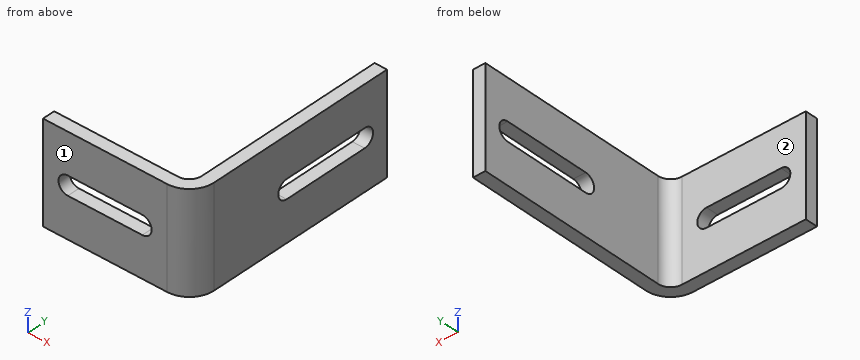
Autodesk Inventor part; units mm, degrees
ref_plane "YZ Plane" through (0, 0, 0) normal (1, 0, 0) x (0, 1, 0)
ref_plane "XZ Plane" through (0, 0, 0) normal (0, 1, 0) x (-1, 0, 0)
ref_plane "XY Plane" through (0, 0, 0) normal (0, 0, 1) x (1, 0, 0)
sketch "スケッチ1" plane through (0, 0, 0) normal (0, 1, 0) x (-1, 0, 0)
  line L0 (-10, 8) -> (10, 8)
  line L1 (10, 8) -> (10, -8)
  line L2 (10, -8) -> (-10, -8)
  line L3 (-10, -8) -> (-10, 8)
  line L4 (-10, 8) -> (10, -8) construction
  line L5 (10, 8) -> (-10, -8) construction
  point P0 (0, 0)
  dimension "d0" = 20
  dimension "d1" = 16
extrude "プレート1" add sketch "スケッチ1" along normal blind 2
sketch "スケッチ2" plane through (12, 4, -8) normal (1, 0, 0) x (0, 1, 0)
  line L0 (0, 16) -> (0, 0)
  line L1 (0, 0) -> (31, 0)
  line L2 (31, 0) -> (31, 16)
  line L3 (31, 16) -> (0, 16)
edge flange "フランジ1" height 35 angle 90 thickness 2 bend radius 2 thickness toward (1, 0, 0) relief tear relief width 2 relief depth 1 edges at (10, 2, 0) wall of the first edge with corners at (12, 4, 8) (12, 4, -8) (12, 35, -8) (12, 35, 8)
bend "曲げ1"
corner "コーナー1"
sketch "スケッチ3" plane through (14, 35, 8) normal (1, 0, 0) x (0, 0, -1)
  line L0 (6.5, -4) -> (6.5, -18)
  arc A0 (6.5, -18) -> (9.5, -18) centre (8, -18) ccw
  line L1 (9.5, -18) -> (9.5, -4)
  arc A1 (9.5, -4) -> (6.5, -4) centre (8, -4) ccw
  line L2 (16, 0) -> (16, -31)
  line L3 (0, 0) -> (16, 0)
  point P0 (8, -35)
  point P1 (8, 0)
  dimension "d19" = 1.5
extrude "押し出し1" cut sketch "スケッチ3" against normal blind 10
sketch "スケッチ4" plane through (0, 2, 0) normal (0, 1, 0) x (1, 0, 0)
  line L0 (-6, -1.5) -> (6, -1.5)
  arc A0 (6, -1.5) -> (6, 1.5) centre (6, 0) ccw
  line L1 (6, 1.5) -> (-6, 1.5)
  arc A1 (-6, 1.5) -> (-6, -1.5) centre (-6, 0) ccw
  line L2 (-10, -8) -> (-10, 8)
  line L3 (10, 8) -> (10, -8)
  point P0 (0, 0)
  dimension "d23" = 4
  dimension "d24" = 4
  dimension "d25" = 1.5
extrude "押し出し2" cut sketch "スケッチ4" against normal blind 10
equation "\"d2\" = Thickness"
equation "\"d3\" = BendReliefWidth"
equation "\"d4\" = BendReliefDepth"
equation "\"d5\" = MinimumRemnant"
equation "\"d6\" = TransitionRadius"
equation "\"d9\" = BendRadius"
equation "\"d10\" = CornerReliefSize"
equation "\"d11\" = GapSize"
equation "\"d12\" = JacobiRadiusSize"
equation "\"BendRadius\" = Thickness"
equation "\"BendReliefWidth\" = Thickness"
equation "\"BendReliefDepth\" = 0.5 * Thickness"
equation "\"CornerReliefSize\" = 4 * Thickness"
equation "\"MinimumRemnant\" = 2 * Thickness"
equation "\"TransitionRadius\" = BendRadius"
equation "\"JacobiRadiusSize\" = BendRadius"
equation "\"GapSize\" = Thickness"
properties part number "keyL_large" material "アルミニウム 6061"
Could you check a few things on this model? Use its own coordinates, in mm. Face numbers are marked on the shaded views. A direction names the side the tool comes from. Give positions to 0.01 mm unless a question says otherwise; leave off trailing zeros. Write each loop counter-clockwise with the first axis right and the second up, starting at its lowest first coordinate (ties: lowest second). Pieces come first, ordered by that corner, then holes. Notation, with made-up numbers: (77.25, 85) - (96.25, 85) arc R10 cw to (96.25, 94) - close; hole circle Ø4 at (89, -2). An arc over 180 degrees is marked (long way). One line per item, written item: value. Start each with the question number.
Item 1: Imagine slicing it at A-A, the plane z = 0. List the corners of the cut face in (x, y) for me.
Item 2: I'm going to push flat-ended pins straight in: pin 1 (3 mm diameter, centred on x = -1, z = -4.5, fed in from -Y); pin 2 (6 mm diameter, centred on x = 1.5, z = 3, fed in from +Y); pin 3 (3 mm diameter, centred on y = 12, z = -4.5, fed in from -X). Where does each tip first touch, or does it pass through?
Item 3: Imagine slicing it at C-C, the plane y = 22. List the corners of the cut face in (x, z) for me, and give its area (3 significant figures).
Item 4: Imagine slicing it at B-B, the plane x = -1.75. List the corners of the cut face in (y, z) for me, and give its area (3 significant figures).
Item 5: Which directions (+Z, -Z, +X, -X, +Y, -Y) give clear straight access to the entire face, cutting with the end or side of a thin tool? Please do the marked faces 1 and 2.
Item 6: Please list where these lines run through material, in increasing order: line 1 (Z direction, x = 13.25, y = 19); line 2 (X direction, y = 23, z = 2.25); line 3 (Y direction, x = 7, z = -3.5). Write a range as from..to.
Item 7: Imagine slicing it at D-D, the plane z = 5.5. List the corners of the cut face in (x, y) for me, and give its area (3 significant figures).
Geometry says:
1. outline: (-10, 0) - (-7.5, 0) - (-7.5, 2) - (-10, 2) - close; (7.5, 0) - (10, 0) arc R4 ccw to (14, 4) - (14, 15.5) - (12, 15.5) - (12, 4) arc R2 cw to (10, 2) - (7.5, 2) - close; (12, 32.5) - (14, 32.5) - (14, 35) - (12, 35) - close
2. pin 1: y = 0
2. pin 2: y = 2
2. pin 3: x = 12
3. outline: (12, -8) - (14, -8) - (14, -1.5) - (12, -1.5) - close; (12, 1.5) - (14, 1.5) - (14, 8) - (12, 8) - close
3. area: 26.0 mm^2
4. outline: (0, -8) - (2, -8) - (2, -1.5) - (0, -1.5) - close; (0, 1.5) - (2, 1.5) - (2, 8) - (0, 8) - close
4. area: 26.0 mm^2
5. face 1: +Z, -Z, +X, -X, -Y
5. face 2: +Z, -Z, -X, +Y
6. line 1: -8..-1.5, 1.5..8
6. line 2: 12..14
6. line 3: 0..2
7. outline: (-10, 0) - (10, 0) arc R4 ccw to (14, 4) - (14, 35) - (12, 35) - (12, 4) arc R2 cw to (10, 2) - (-10, 2) - close
7. area: 111 mm^2
